Read the model definition and answer for the solid it produces. Units are mm, in the model's axes. Coordinates: 2 decimals unless noted, no trailing zeros. Write each loop counter-clockwise with the first axis right and the second up, starting at its lowest first coordinate (ties: lowest second). Pieces come first, ordered by that corner, then holes. Notation, with made-up numbers: (25.5, 0) -> (48.5, 0) arc R28 cw to (48.5, 33) -> close; hole circle Ø1 at (62.5, 13). An arc over 180 degrees is marked (long way). Answer in a Markdown table with one row per item. Add a question column.
Item 1: Section D-D on z = 35 is taken. Write down the section's boundary in (x, y).
Item 2: Section B-B on y = -5 is taken. Write down the section's boundary in (x, z), then the cut area to 3 significant figures.
Item 3: Section A-A on z = 65 is taken. Write down the section's boundary in (x, y).
Item 4: Given pin 1 Ø1 at (y, z) = (-8.5, 80) entering from -X; pin 2 Ø4 at (x, z) = (0, 0) entering from +Y, each flat-ended and moving along its own axis, determine where each tip first touches the part or whether it passes through.
Item 5: Section C-C on x = 18 is taken. Write down the section's boundary in (y, z), then the cut area to 3 significant figures.
Item 6: Straight lines are drawn through the part: line 1 (X direction, y = -2.5, z = 67); line 2 (Y direction, x = 14, z = 132); line 3 (X direction, y = -9.7, z = 140). For each, find the intervals that lie inside material, in ascending order. Write a range as from..to.
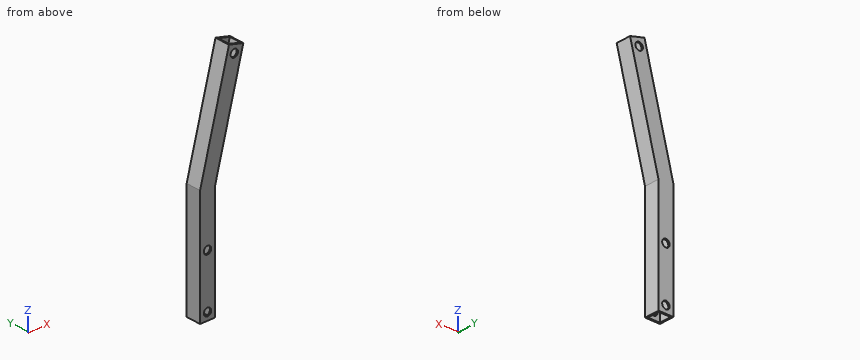
```python
from build123d import *

# Parameters (mm, degrees)
PAD_DEPTH    = 10
THICKNESS_T  = -1
SKETCH001_R  = 2.5
POCKET_DEPTH = 10.001


with BuildPart() as part:
    # Sketch → Pad (new body)
    with BuildSketch(Plane.XZ):
        Polygon((-5, -5), (-5, 70.632568), (14.402741, 146.08767), (24.08767, 143.597259), (5, 69.367432), (5, -5), align=None)
    extrude(amount=PAD_DEPTH)

    # Thickness
    thickness_openings = [part.faces().sort_by_distance(p)[0] for p in [
        (19.245205, -5, 144.842465),
        (0, -5, -5),
    ]]
    offset(amount=THICKNESS_T, openings=thickness_openings)

    # Sketch001 (on Face6 of Thickness) → Pocket (cut, through all)
    with BuildSketch(Plane.XZ.offset(10)):
        with Locations((18, 140)):
            Circle(SKETCH001_R)
        Circle(SKETCH001_R)
        with Locations((0, 35)):
            Circle(SKETCH001_R)
    extrude(amount=-POCKET_DEPTH, mode=Mode.SUBTRACT)


solid = part.part
```
Results below:
| question | item | result |
|---|---|---|
| 1 | outline | (-5, -10) -> (-2.5, -10) -> (-2.5, -9) -> (-4, -9) -> (-4, -1) -> (-2.5, -1) -> (-2.5, 0) -> (-5, 0) -> close; (2.5, -10) -> (5, -10) -> (5, 0) -> (2.5, 0) -> (2.5, -1) -> (4, -1) -> (4, -9) -> (2.5, -9) -> close |
| 2 | outline | (-5, -5) -> (-4, -5) -> (-4, 70.51) -> (15.37, 145.84) -> (14.4, 146.09) -> (-5, 70.63) -> close; (4, -5) -> (5, -5) -> (5, 69.37) -> (24.09, 143.6) -> (23.12, 143.85) -> (4.03, 69.62) arc R1 ccw to (4, 69.37) -> close |
| 2 | area | 305 mm2 |
| 3 | outline | (-5, -10) -> (5, -10) -> (5, 0) -> (-5, 0) -> close; hole (-4, -9) -> (4, -9) -> (4, -1) -> (-4, -1) -> close |
| 4 | pin 1 | stops at x = -2.72 |
| 4 | pin 2 | passes through |
| 5 | outline | (-10, 119.92) -> (0, 119.92) -> (0, 137.5) -> (-1, 137.5) -> (-1, 123.94) -> (-9, 123.94) -> (-9, 137.5) -> (-10, 137.5) -> close; (-10, 142.5) -> (-9, 142.5) -> (-9, 145.16) -> (-10, 145.16) -> close; (-1, 142.5) -> (0, 142.5) -> (0, 145.16) -> (-1, 145.16) -> close |
| 5 | area | 72.6 mm2 |
| 6 | line 1 | x = -5..-4, 4..5 |
| 6 | line 2 | y = -10..-9, -1..0 |
| 6 | line 3 | x = 12.84..15.5, 20.5..23.16 |
